For this review, take the finished solid that the model builds, in its own axes (mm). Give positions to 0.01 mm unless a question says otherwise; leave off trailing zeros. Loops run counter-clockwise (first coordinate to the right, second up) from the corner with the lowest first, then second, coordinate; pieces in that order, holes last. Notation, with made-up numbers: (16, 81.5) - (53, 81.5) arc R5 cw to (53, 89.5) - close; hole circle Ø4 at (9.25, 81). An arc over 180 degrees is marked (long way). Answer in a Markdown table with one row per item.
Autodesk Inventor part; units mm, degrees
ref_plane "YZ Plane" through (0, 0, 0) normal (1, 0, 0) x (0, 1, 0)
ref_plane "XZ Plane" through (0, 0, 0) normal (0, 1, 0) x (-1, 0, 0)
ref_plane "XY Plane" through (0, 0, 0) normal (0, 0, 1) x (1, 0, 0)
sketch "Sketch1" plane through (0, 0, 0) normal (0, 0, 1) x (1, 0, 0)
  line L0 (-47.2018, -34.166) -> (42.7982, -34.166)
  line L1 (42.7982, -34.166) -> (42.7982, 35.834)
  line L2 (42.7982, 35.834) -> (-47.2018, 35.834)
  line L3 (-47.2018, 35.834) -> (-47.2018, -34.166)
  circle A0 centre (-42.2305, -29.3992) radius 2.5544
  point P0 (0, 0)
  dimension "d0" = 90
  dimension "d1" = 70
extrude "Extrusion1" add sketch "Sketch1" along normal blind 1 contours L3 L2 L1 L0 | A0
extrude "Extrusion2" add sketch "Sketch1" along normal blind 10 contours A0
properties part number "protoboard"
1. Clearance check with flat-ended pins moving along their axes: pin 1 (4 mm diameter, centred on x = 20, y = -9, fed in from +Z); pin 2 (2 mm diameter, centred on y = -17.5, z = 1.5, fed in from +X). State where each tip first meets the part, or that it passes through.
Values:
| item | result |
|---|---|
| pin 1 | stops at z = 1 |
| pin 2 | stops at x = 42.8 |
2. Mouldability with a two-part tool opening along Y and no side actions: class faces 1 (the face through (-42, -29, 10)), 2 (the face through (-44.782, -29.512, 5.437)) as released by +Y, released by -Y, zero draft, split by the parting line, or undercut.
Values:
| item | result |
|---|---|
| face 1 | zero draft |
| face 2 | split by the parting line |
3. We need section A-A, the plane y = 28. Give the boundary of the cut face in (x, z), and give its area (3 significant figures).
Values:
| item | result |
|---|---|
| outline | (-47.2, 0) - (42.8, 0) - (42.8, 1) - (-47.2, 1) - close |
| area | 90.0 mm^2 |
4. We need section B-B, the plane x = 33. Give the boundary of the cut face in (y, z), and give its area (3 significant figures).
Values:
| item | result |
|---|---|
| outline | (-34.17, 0) - (35.83, 0) - (35.83, 1) - (-34.17, 1) - close |
| area | 70.0 mm^2 |
5. Wall thickness on line 1 (Z direction, x = 0.5, y = -13); line 2 (Y direction, x = -42.5, z = 1.25); line 3 (Y direction, x = -43, z = 6): over which ranges is each line inside the solid? List them lowest first. Write a range as [from, to].
Values:
| item | result |
|---|---|
| line 1 | z = [0, 1] |
| line 2 | y = [-31.94, -26.86] |
| line 3 | y = [-31.83, -26.96] |
6. We need section C-C, the plane z = 8.75. Give the boundary of the cut face in (x, y), and give its area (3 significant figures).
Values:
| item | result |
|---|---|
| outline | circle Ø5.11 at (-42.23, -29.4) |
| area | 20.5 mm^2 |
